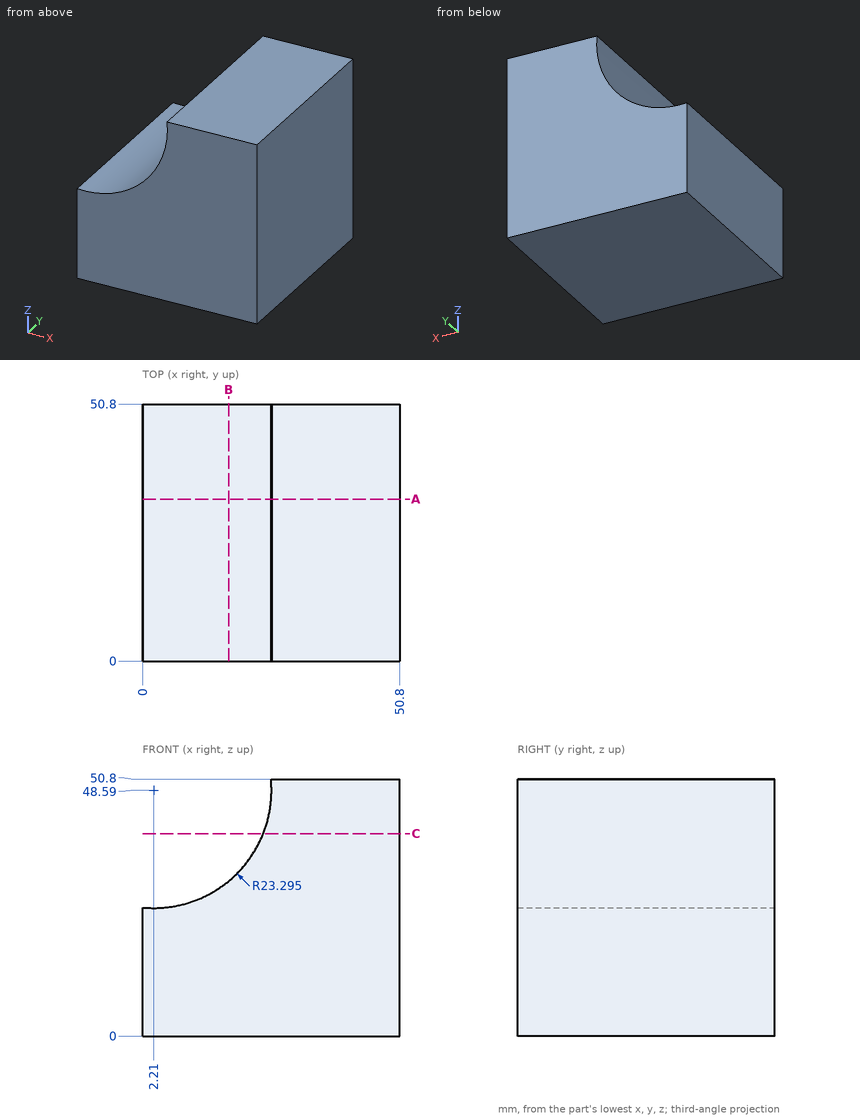
Job drawing, mm, ordinate dimensions from the low corner. One solid piece. Round coordinates to 2 decimals unless told otherwise and drop trailing zeros. Write each loop counter-clockwise with the first axis right and the second up, starting at its lowest first coordinate (ties: lowest second). Pieces come first, ordered by that corner, then holes. Notation, with made-up numbers: (84.25, 75) -> (133.25, 75) arc R28 cw to (133.25, 107) -> close; hole circle Ø2 at (-30.75, 66). An arc over 180 degrees is marked (long way). Answer as a JSON object with one key per item and string values.
(1) Pin check, flat tips, straight feed: P1, Ø6, axis at y = 26.5, z = 33.5, coming from the -X side; P2, Ø4, axis at y = 43.5, z = 41, coming from the -X side; P3, Ø3, axis at y = 16, z = 29.5, coming from the -X side. Stop position of each tip, or through.
Reported:
{"P1": "stops at x = 16.89", "P2": "stops at x = 23.44", "P3": "stops at x = 13.11"}
(2) Band-saw the part on B-B, the plane x = 17. List the corners of the cut face in (y, z).
Reported:
{"outline": "(0, 0) -> (50.8, 0) -> (50.8, 30.59) -> (0, 30.59) -> close"}
(3) Probe probe 1 along X at (y, z) = (11, 46.5); probe 2 along X at (y, z) = (15, 48); probe 3 along Z at (x, y) = (4.5, 43). List the from-to ranges inside material, lowest first. Write a range as [from, to].
Reported:
{"probe 1": "x = [25.41, 50.8]", "probe 2": "x = [25.5, 50.8]", "probe 3": "z = [0, 25.41]"}
(4) Band-saw the part on A-A, the plane y = 32. List the corners of the cut face in (x, z) (3 decimals).
Reported:
{"outline": "(0, 0) -> (50.8, 0) -> (50.8, 50.8) -> (25.4, 50.8) arc R23.295 cw to (0, 25.4) -> close"}
(5) Band-saw the part on C-C, the plane z = 40. List the corners of the cut face in (x, y), then the cut area to 3 significant figures.
Reported:
{"outline": "(23.86, 0) -> (50.8, 0) -> (50.8, 50.8) -> (23.86, 50.8) -> close", "area": "1,370 mm^2"}
